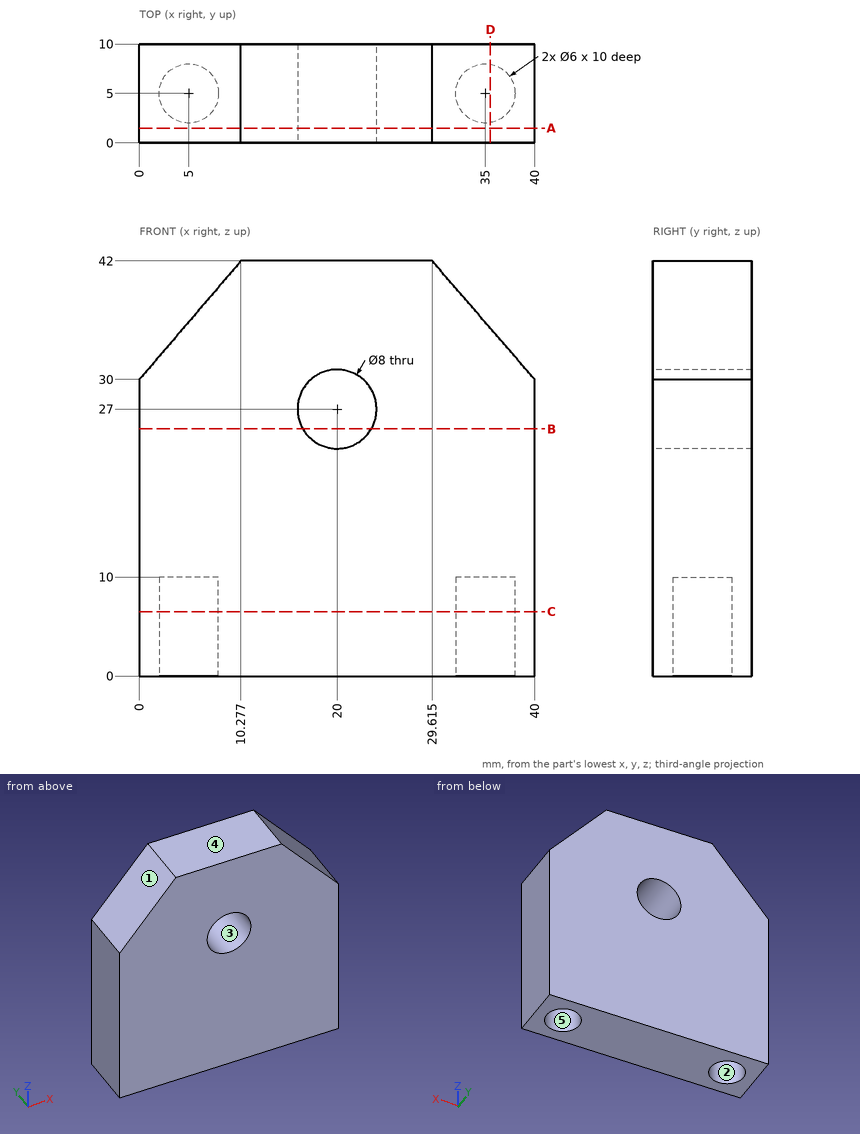
For this review, use the dimensioned drawing (mm, ordinates from the lowest corner) and the shaded views. A direction names the side the tool comes from. Give positions to 0.01 mm unless a question says otherwise; leave off trailing zeros. Write each loop counter-clockwise with the first axis right and the second up, starting at its lowest first coordinate (ties: lowest second). Pieces come first, ordered by that corner, then holes. Notation, with made-up numbers: M 78.5,62 L 115.5,62 A19 ccw 115.5,91 Z; hole C 37.5,63 d11. An arc over 180 degrees is marked long. Answer as a JSON object with one key per item and string values. Group by question number.
1) We need section A-A (y = 1.5). Give the boundary of the cut face in (x, z) (3 decimals).
2) Tool access review of the marked faces 4 and 5: name each direction out of +Z, -Z, +X, -X, +Y, -Y from which nothing blocks a thin tool from reaching the whole face with its end or side.
3) We need section B-B (z = 25). Give the boundary of the cut face in (x, y).
4) Clearance check with flat-ended pins moving along their axes: pin 1 Ø6.5 at (x, z) = (20, 27) entering from -Y; pin 2 Ø3 at (x, y) = (5, 4) entering from -Z. State where each tip first meets the part, or that it passes through.
5) Mouldability with a two-part tool opening along Z and no side actions: class the marked faces 1, 2 and 3 as released by +Z, released by -Z, zero draft, split by the parting line, or undercut.
6) We need section C-C (z = 6.5). Give the boundary of the cut face in (x, y), and give its area (3 significant figures).
7) We need section D-D (x = 35.5). Give the boundary of the cut face in (y, z), and give its area (3 significant figures).
8) For line 1 along X through (y, z) = (5, 2.5); line 2 along Z through (x, y) = (20, 8.25); line 3 along X through (y, z) = (5.75, 9.5) (1 decimal), list the stretches that pass through material, from the lowest coordinate up.
Answer key:
{
 "1": {"outline": "M 0,0 L 40,0 L 40,30 L 29.615,42 L 10.277,42 L 0,30 Z; hole C 20,27 d8"},
 "2": {"face 4": "+Z, +X, -X, +Y, -Y", "face 5": "-Z"},
 "3": {"outline": "M 0,0 L 16.54,0 L 16.54,10 L 0,10 Z; M 23.46,0 L 40,0 L 40,10 L 23.46,10 Z"},
 "4": {"pin 1": "passes through", "pin 2": "stops at z = 10"},
 "5": {"face 1": "released by +Z", "face 2": "zero draft", "face 3": "undercut"},
 "6": {"outline": "M 0,0 L 40,0 L 40,10 L 0,10 Z; hole C 5,5 d6; hole C 35,5 d6", "area": "343 mm²"},
 "7": {"outline": "M 0,0 L 2.04,0 L 2.04,10 L 7.96,10 L 7.96,0 L 10,0 L 10,35.2 L 0,35.2 Z", "area": "293 mm²"},
 "8": {"line 1": "x = 0 to 2, 8 to 32, 38 to 40", "line 2": "z = 0 to 23, 31 to 42", "line 3": "x = 0 to 2.1, 7.9 to 32.1, 37.9 to 40"}
}
